Can you work these out from the drawing? Everything is in mm from the part's minimum corner. Give positions to 0.01 mm unless a question says otherwise; leave off trailing zeros. Order: outer loops, then holes, each group sorted by start corner. A loop starts at its lowest first (then second) coordinate and runs counter-clockwise, first axis right, second up. Notation, with made-up numbers: (35, 0) - (52, 0) arc R20 cw to (52, 11) - close; hole circle Ø10 at (46, 62.5). An arc over 180 degrees is marked (long way). One line per question, with ' | ' between items.
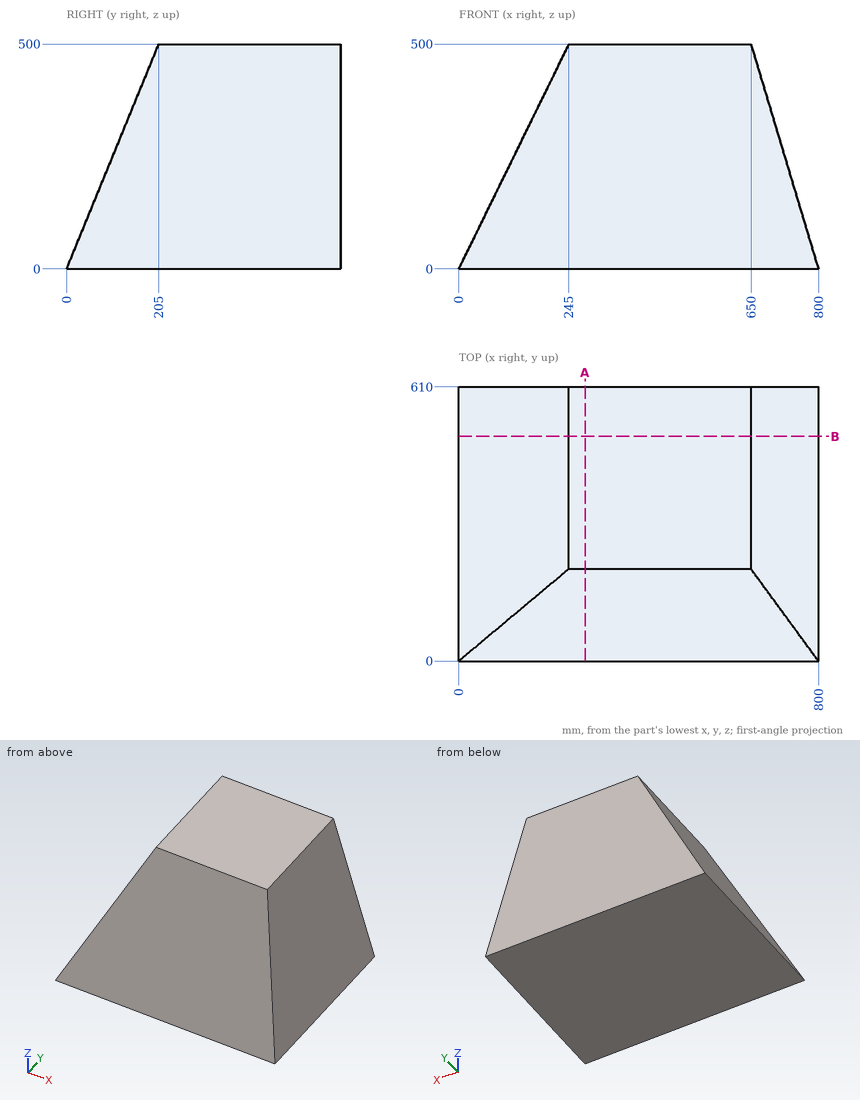
1) Please list where these lines run through material, in increasing order: L1, parallel to Z at x = 232, y = 46; L2, parallel to Y at x = 422, z = 409.5 (3 decimals); L3, parallel to Z at x = 639, y = 105.5.
Model answer:
L1: z = 0 to 112.2 | L2: y = 167.895 to 610 | L3: z = 0 to 257.32
2) I want a section at B-B (y = 500). List the corners of the cut face in (x, z) for me.
Model answer:
outline: (0, 0) - (800, 0) - (650, 500) - (245, 500) - close
3) I want a section at A-A (x = 281). List the corners of the cut face in (y, z) for me, plus the area to 3 significant figures.
Model answer:
outline: (0, 0) - (610, 0) - (610, 500) - (205, 500) - close | area: 254,000 mm2
4) I'm going to push flat-ended pins straight in: P1, Ø6, axis at x = 121.5, z = 157, coming from the -Y side; P2, Ø5, axis at x = 447.5, z = 145.5, coming from the -Y side; P3, Ø2, axis at y = 119.5, z = 89, coming from the -X side. Where does each tip first touch, or does it pass through?
Model answer:
P1: stops at y = 63.14 | P2: stops at y = 58.63 | P3: stops at x = 43.12
